Can you work these out from the model? Positions are in its coordinate system, mm. A direction names the side the tool comes from. Coordinates: 2 decimals unless noted, no trailing zeros. Order: outer loops, then holes, each group sorted by start corner. A loop starts at its lowest first (then second) coordinate and runs counter-clockwise, first axis right, second up. Notation, with made-up numbers: (-12.75, 1) -> (3.25, 1) arc R4 cw to (3.25, 7) -> close; hole circle Ø6 at (-5.5, -13.75). An arc over 180 degrees is marked (long way). Write item = value, one per line.
```python
from build123d import *

# Parameters (mm, degrees)
BOSS_EXTRUDE1_DEPTH = 2.55
BOSS_EXTRUDE2_DEPTH = 1.075


with BuildPart() as part:
    # Sketch1 → Boss-Extrude1 (new body, symmetric)
    with BuildSketch(Plane.XY):
        with BuildLine():
            ThreePointArc((3.727642468, 0.408878505), (0, 3.75), (-3.727642468, 0.408878505))
            ThreePointArc((-3.727642468, 0.408878505), (-3.75, 0), (-3.727642468, -0.408878505))
            ThreePointArc((-3.727642468, -0.408878505), (0, -3.75), (3.727642468, -0.408878505))
            ThreePointArc((3.727642468, -0.408878505), (3.744406445, -0.204744652), (3.75, 0))
            ThreePointArc((3.75, 0), (3.744406445, 0.204744652), (3.727642468, 0.408878505))
        make_face()
        with BuildLine():
            Line((0.25, -1.984313483), (0.25, -2.5))
            Line((0.25, -2.5), (-0.25, -2.5))
            Line((-0.25, -2.5), (-0.25, -1.984313483))
            ThreePointArc((-0.25, -1.984313483), (-2, 0), (-0.25, 1.984313483))
            Line((-0.25, 1.984313483), (-0.25, 2.5))
            Line((-0.25, 2.5), (0.25, 2.5))
            Line((0.25, 2.5), (0.25, 1.984313483))
            ThreePointArc((0.25, 1.984313483), (1.5, 1.322875656), (2, 0))
            ThreePointArc((2, 0), (1.5, -1.322875656), (0.25, -1.984313483))
        make_face(mode=Mode.SUBTRACT)
    extrude(amount=BOSS_EXTRUDE1_DEPTH, both=True)

    # Sketch2 → Boss-Extrude2 (add, symmetric)
    with BuildSketch(Plane.XY):
        with BuildLine():
            Line((-1.988075983, 16.268068536), (-3.727642468, 0.408878505))
            ThreePointArc((-3.727642468, 0.408878505), (0, 3.75), (3.727642468, 0.408878505))
            Line((3.727642468, 0.408878505), (1.988075983, 16.268068536))
            ThreePointArc((1.988075983, 16.268068536), (0, 18.05), (-1.988075983, 16.268068536))
        make_face()
        with BuildLine():
            ThreePointArc((3.727642468, -0.408878505), (0, -3.75), (-3.727642468, -0.408878505))
            Line((-3.727642468, -0.408878505), (-1.988075983, -16.268068536))
            ThreePointArc((-1.988075983, -16.268068536), (0, -18.05), (1.988075983, -16.268068536))
            Line((1.988075983, -16.268068536), (3.727642468, -0.408878505))
        make_face()
    extrude(amount=BOSS_EXTRUDE2_DEPTH, both=True)


solid = part.part
```
Item 1: I want a section at C-C, the plane z = 1.65. Please give me the cut outline in (x, y), plus the area to 3 significant figures.
A:
outline = circle Ø7.5 at (0, 0); hole (-0.25, -2.5) -> (0.25, -2.5) -> (0.25, -1.98) arc R2 ccw to (0.25, 1.98) -> (0.25, 2.5) -> (-0.25, 2.5) -> (-0.25, 1.98) arc R2 ccw to (-0.25, -1.98) -> close
area = 31.1 mm2
Item 2: I want a section at A-A, the plane z = 0.2. Please give me the cut outline in (x, y), plus the area to 3 significant figures.
A:
outline = (-3.73, -0.41) -> (-1.99, -16.27) arc R2 ccw to (1.99, -16.27) -> (3.73, -0.41) arc R3.75 ccw to (3.73, 0.41) -> (1.99, 16.27) arc R2 ccw to (-1.99, 16.27) -> (-3.73, 0.41) arc R3.75 ccw to start; hole (-0.25, -2.5) -> (0.25, -2.5) -> (0.25, -1.98) arc R2 ccw to (0.25, 1.98) -> (0.25, 2.5) -> (-0.25, 2.5) -> (-0.25, 1.98) arc R2 ccw to (-0.25, -1.98) -> close
area = 185 mm2
Item 3: I want a section at B-B, the plane x = -1.5. Please give me the cut outline in (y, z) (3 decimals), plus the area to 3 significant figures.
A:
outline = (-17.373, -1.075) -> (-3.437, -1.075) -> (-3.437, -2.55) -> (-1.323, -2.55) -> (-1.323, 2.55) -> (-3.437, 2.55) -> (-3.437, 1.075) -> (-17.373, 1.075) -> close; (1.323, -2.55) -> (3.437, -2.55) -> (3.437, -1.075) -> (17.373, -1.075) -> (17.373, 1.075) -> (3.437, 1.075) -> (3.437, 2.55) -> (1.323, 2.55) -> close
area = 81.5 mm2
Item 4: If we mould it in two halves opening along Y, with no side actions, what happens to faces 3 (the flat face through (2.846, -8.449, 0.015)), 4 (the cylindrical face through (0.04, 18.05, -0.02)), 5 (the cylindrical face through (-2, 0, 0))? For each: pulls with the +Y half, pulls with the -Y half, needs draft (parallel to the pull), parting line crosses it, or undercut.
A:
face_3 = pulls with the -Y half
face_4 = pulls with the +Y half
face_5 = undercut
Item 5: I want a section at D-D, the plane x = -3. Please give me the cut outline in (y, z) (3 decimals).
A:
outline = (-7.043, -1.075) -> (-2.25, -1.075) -> (-2.25, -2.55) -> (2.25, -2.55) -> (2.25, -1.075) -> (7.043, -1.075) -> (7.043, 1.075) -> (2.25, 1.075) -> (2.25, 2.55) -> (-2.25, 2.55) -> (-2.25, 1.075) -> (-7.043, 1.075) -> close
Item 6: If I drill on probe 1 along Z at (x, y) = (2.5, 4.5) (3 decimals); probe 2 along Y at (x, z) = (-1.5, -1.6); probe 3 along Y at (x, z) = (0.5, 0.65), over which ranges is the centre line in solid material (lowest first)?
A:
probe_1 = -1.075 to 1.075
probe_2 = -3.44 to -1.32, 1.32 to 3.44
probe_3 = -17.99 to -1.94, 1.94 to 17.99
Item 7: I'm going to push flat-ended pins straight in: P1, Ø4, axis at x = 3, y = 11.5, coming from the -Z side (3 decimals); P2, Ø3, axis at y = -13, z = 0, coming from the +X side; P3, Ø0.6, axis at y = 2.5, z = 1, coming from the +X side. Where does each tip first touch, or does it pass through?
A:
P1 = -1.075
P2 = 2.51
P3 = 3.53
Item 8: For faces 1 (the cylindrical face through (2, 0, 0)), 2 (the flat face through (2.87, 8.23, -0.02)), which set-ups out of +Z, -Z, +X, -X, +Y, -Y let a thin tool reach every point of the face, with its end or its side?
A:
face_1 = +Z, -Z
face_2 = +Z, -Z, +X, +Y
